Could you check a few things on this drawing? It's one solid part, dimensions in mm from its lowest x, y, z. A direction names the side the tool comes from. Give positions to 0.01 mm unless a question says otherwise; leave off trailing zeros. Order: outer loops, then holes, each group sorted by start corner. A loop starts at its lowest first (then second) coordinate and runs counter-clockwise, first axis right, second up. Notation, with made-up numbers: M 77,-26.5 L 104,-26.5 A19 cw 104,-11.5 Z; hole C 50,52 d4. An arc over 180 degrees is marked long. Return JSON: item names as keys, results as strings. Group by question number.
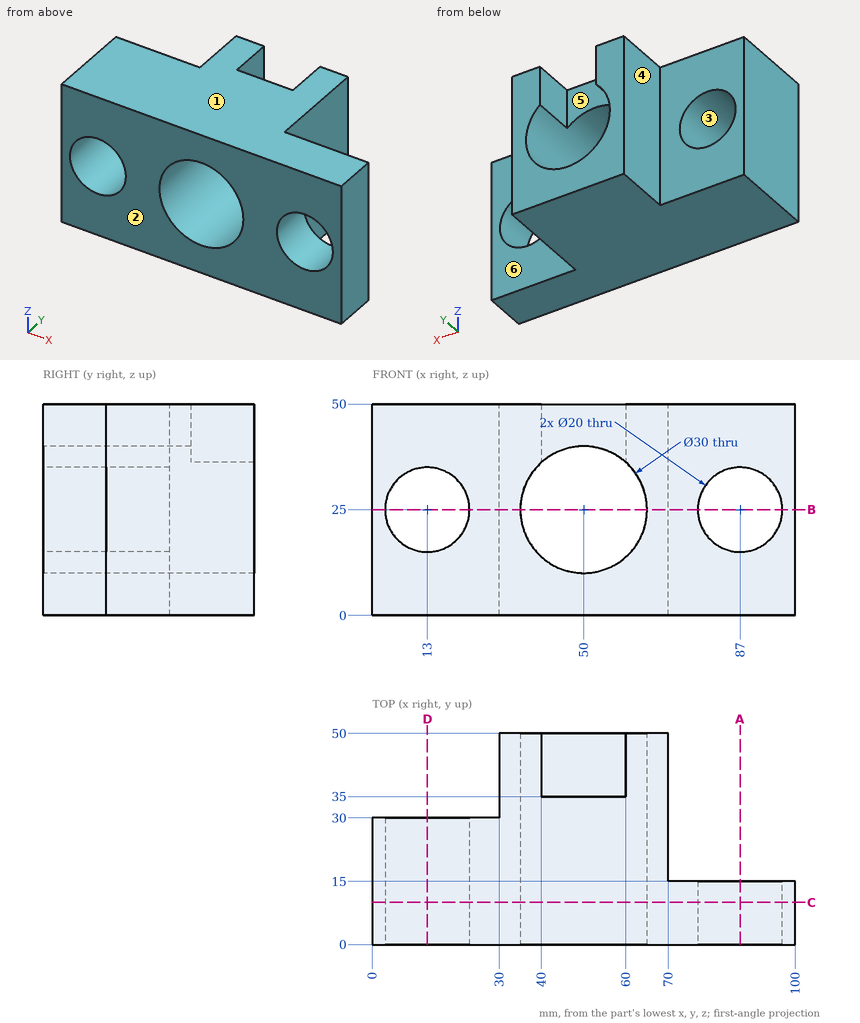
1. Imagine slicing it at C-C, the plane y = 10. Please give me the cut outline in (x, z), plus the area to 3 significant figures.
2. Imagine slicing it at D-D, the plane x = 13. Please give me the cut outline in (y, z), plus the area to 3 significant figures.
3. Which directions (+Z, -Z, +X, -X, +Y, -Y) give clear straight access to the entire face, cutting with the end or side of a thin tool? Please do the marked faces 4, 5 and 6.
4. If we mould it in two halves opening along Z, with no side actions, what happens to the marked faces 1, 2 and 3? For each: pulls with the +Z half, pulls with the -Z half, needs draft (parallel to the pull), parting line crosses it, or undercut.
5. Imagine slicing it at A-A, the plane x = 87. Please give me the cut outline in (y, z), plus the area to 3 significant figures.
6. Imagine slicing it at B-B, the plane z = 25. Please give me the cut outline in (x, y), plus the area to 3 significant figures.
7. I need wall thicknesses on L1, parallel to X at y = 47, z = 44; L2, parallel to Z at x = 50, y = 27.5; L3, parallel to Z at x = 87, y = 4.25. Which ranges of each line are inside material? Lowest first, please. Write a range as from..to.
8. For pin 1 (24 mm diameter, centred on x = 85, z = 27, fed in from +Y); pin 2 (7 mm diameter, centred on x = 53, z = 40.5, fed in from +Y); pin 3 (11 mm diameter, centred on y = 42, z = 42, fed in from -X), each with a flat end and sliding along its axis, tell me the tip position at first contact or that it passes through.
Values:
{
 "1": {"outline": "M 0,0 L 100,0 L 100,50 L 0,50 Z; hole C 13,25 d20; hole C 50,25 d30; hole C 87,25 d20", "area": "3,660 mm²"},
 "2": {"outline": "M 0,0 L 30,0 L 30,15 L 0,15 Z; M 0,35 L 30,35 L 30,50 L 0,50 Z", "area": "900 mm²"},
 "3": {"face 4": "+Z, -Z, -X, +Y", "face 5": "+Z, +Y", "face 6": "+Z, -Z, +X, +Y"},
 "4": {"face 1": "pulls with the +Z half", "face 2": "needs draft", "face 3": "undercut"},
 "5": {"outline": "M 0,0 L 15,0 L 15,15 L 0,15 Z; M 0,35 L 15,35 L 15,50 L 0,50 Z", "area": "450 mm²"},
 "6": {"outline": "M 0,0 L 3,0 L 3,30 L 0,30 Z; M 23,0 L 35,0 L 35,50 L 30,50 L 30,30 L 23,30 Z; M 65,0 L 77,0 L 77,15 L 70,15 L 70,50 L 65,50 Z; M 97,0 L 100,0 L 100,15 L 97,15 Z", "area": "950 mm²"},
 "7": {"L1": "x = 30..40, 60..70", "L2": "z = 0..10, 40..50", "L3": "z = 0..15, 35..50"},
 "8": {"pin 1": "stops at y = 15", "pin 2": "stops at y = 35", "pin 3": "stops at x = 30"}
}
